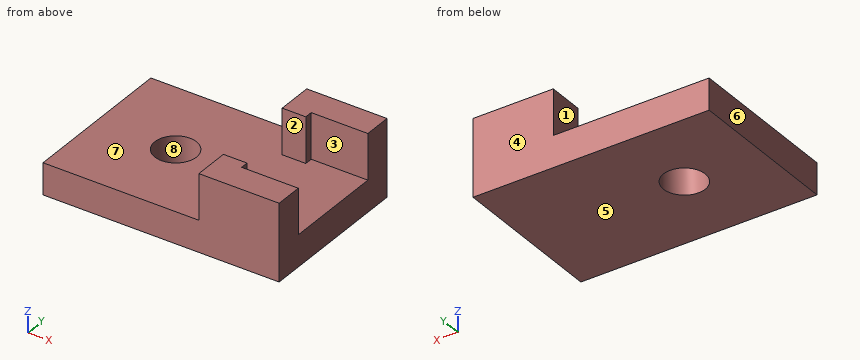
from build123d import *

# Parameters (mm, degrees)
SKETCH1_W           = 30
SKETCH1_H           = 20
BOSS_EXTRUDE1_DEPTH = 4
SKETCH2_R           = 2.65
CUT_EXTRUDE1_DEPTH  = 37.276714294
BOSS_EXTRUDE2_DEPTH = 5.8


with BuildPart() as part:
    # Sketch1 → Boss-Extrude1 (new body)
    with BuildSketch(Plane.XY):
        with Locations((15, -10)):
            Rectangle(SKETCH1_W, SKETCH1_H)
    extrude(amount=BOSS_EXTRUDE1_DEPTH)

    # Sketch2 → Cut-Extrude1 (cut, through all)
    with BuildSketch(Plane.XY.offset(4)):
        with Locations((10, -10)):
            Circle(SKETCH2_R)
    extrude(amount=-CUT_EXTRUDE1_DEPTH, mode=Mode.SUBTRACT)

    # Sketch3 → Boss-Extrude2 (add)
    with BuildSketch(Plane.XY.offset(4)):
        Polygon((22.8, -4.55), (22.8, -3.55), (22.8, 0), (19.8, 0), (19.8, -4.55), align=None)
        Polygon((22.8, 0), (22.8, -3.55), (29, -3.55), (30, -3.55), (30, 0), align=None)
        Polygon((22.8, -16.45), (22.8, -15.45), (19.8, -15.45), (19.8, -20), (22.8, -20), align=None)
        Polygon((30, -16.45), (29, -16.45), (22.8, -16.45), (22.8, -20), (30, -20), align=None)
    extrude(amount=BOSS_EXTRUDE2_DEPTH)


solid = part.part
Input: part model. Units: mm. Frame: model coordinates. Face numbers are marked on the shaded views. A direction names the side the tool comes from. Round coordinates to 2 decimals unless told otherwise and drop trailing zeros. Loops run counter-clockwise (first coordinate to the right, second up) from the corner with the lowest first, then second, coordinate; pieces in that order, holes last. Notation, with made-up numbers: (-10, 4) -> (47, 4) arc R21 cw to (47, 43) -> close; hole circle Ø3 at (-34, 38.25). An arc over 180 degrees is marked (long way). Answer as a JSON object with one key per item and string values. Group by question number.
1) Section query C-C on z = 5. Output: boundary loops of the cut face in (x, y).
2) Pin query (flat end, axial travel): pin 1 (1.4 mm diameter, centred on y = -2.5, z = 5.5, fed in from -X); pin 2 (4 mm diameter, centred on x = 5.5, z = 5, fed in from +Y); pin 3 (0.5 mm diameter, centred on y = -4, z = 6, fed in from +X); pin 4 (4 mm diameter, centred on x = 10, y = -10, fed in from +Z). Return the tip coordinate at first contact, or that it passes through.
3) Section query D-D on y = -18.25. Output: boundary loops of the cut face in (x, z), plus the area to 3 significant figures.
4) Reachability of the marked faces 1, 2, 3, 4 and 5 from +Z, -Z, +X, -X, +Y, -Y: full face, straight path, thin tool, end or side. Return the list, or none.
5) Section query B-B on y = -10. Output: boundary loops of the cut face in (x, z).
6) Ray query, L1, parallel to Y at x = 10, z = 1.65; L2, parallel to Y at x = 21, z = 6.5; L3, parallel to Z at x = 9.5, y = -6.5. Return the intervals inside material, ascending.
7) Section query A-A on x = 10. Output: boundary loops of the cut face in (y, z), plus the area to 3 significant figures.
8) Draft query along X for the marked faces 6, 7 and 8. Return one class per face: +X half, -X half, draft (parallel to the pull), parting line (faces both ways), or undercut.
Reply:
{
 "1": {"outline": "(19.8, -20) -> (30, -20) -> (30, -16.45) -> (22.8, -16.45) -> (22.8, -15.45) -> (19.8, -15.45) -> close; (19.8, -4.55) -> (22.8, -4.55) -> (22.8, -3.55) -> (30, -3.55) -> (30, 0) -> (19.8, 0) -> close"},
 "2": {"pin 1": "stops at x = 19.8", "pin 2": "stops at y = 0", "pin 3": "stops at x = 22.8", "pin 4": "passes through"},
 "3": {"outline": "(0, 0) -> (30, 0) -> (30, 9.8) -> (19.8, 9.8) -> (19.8, 4) -> (0, 4) -> close", "area": "179 mm2"},
 "4": {"face 1": "+Z, -X, +Y, -Y", "face 2": "+Z, +X, -X", "face 3": "+Z, +X", "face 4": "+Z, -Z, +X, -X, +Y", "face 5": "-Z, +X, -X, +Y, -Y"},
 "5": {"outline": "(0, 0) -> (7.35, 0) -> (7.35, 4) -> (0, 4) -> close; (12.65, 0) -> (30, 0) -> (30, 4) -> (12.65, 4) -> close"},
 "6": {"L1": "y = -20 to -12.65, -7.35 to 0", "L2": "y = -20 to -15.45, -4.55 to 0", "L3": "z = 0 to 4"},
 "7": {"outline": "(-20, 0) -> (-12.65, 0) -> (-12.65, 4) -> (-20, 4) -> close; (-7.35, 0) -> (0, 0) -> (0, 4) -> (-7.35, 4) -> close", "area": "58.8 mm2"},
 "8": {"face 6": "-X half", "face 7": "draft", "face 8": "undercut"}
}
